from build123d import *

# Parameters (mm, degrees)
SKETCH_W     = 72
SKETCH_H     = 72
PAD_DEPTH    = 1.5
PAD001_DEPTH = 6
SKETCH002_R  = 1.6
POCKET_DEPTH = 7.501
FILLET_R     = 2
CHAMFER_SIZE = 1


with BuildPart() as part:
    # Sketch → Pad (new body)
    with BuildSketch(Plane.XY):
        with Locations((36, -36)):
            Rectangle(SKETCH_W, SKETCH_H)
    extrude(amount=PAD_DEPTH)

    # Sketch001 (on Face6 of Pad) → Pad001 (join)
    with BuildSketch(Plane.XY.offset(1.5)):
        with BuildLine():
            ThreePointArc((0, -8), (5.656854, -5.656854), (8, 0))
            Line((0, 0), (8, 0))
            Line((0, -8), (0, 0))
        make_face()
        with BuildLine():
            ThreePointArc((8, -72), (5.656854, -66.343146), (0, -64))
            Line((0, -72), (0, -64))
            Line((8, -72), (0, -72))
        make_face()
        with BuildLine():
            ThreePointArc((72, -64), (66.343146, -66.343146), (64, -72))
            Line((64, -72), (72, -72))
            Line((72, -72), (72, -64))
        make_face()
        with BuildLine():
            ThreePointArc((64, 0), (66.343146, -5.656854), (72, -8))
            Line((72, -8), (72, 0))
            Line((72, 0), (64, 0))
        make_face()
    extrude(amount=PAD001_DEPTH)

    # Sketch002 (on Face14 of Pad001) → Pocket (cut, through all)
    with BuildSketch(Plane.XY.offset(7.5)):
        with Locations((4, -4)):
            Circle(SKETCH002_R)
        with Locations((68, -4)):
            Circle(SKETCH002_R)
        with Locations((68, -68)):
            Circle(SKETCH002_R)
        with Locations((4, -68)):
            Circle(SKETCH002_R)
    extrude(amount=-POCKET_DEPTH, mode=Mode.SUBTRACT)

    # Fillet
    fillet_edges = [part.edges().sort_by_distance(p)[0] for p in [
        (0, 0, 4.5),
        (72, 0, 4.5),
        (0, -72, 4.5),
        (72, -72, 4.5),
    ]]
    fillet(fillet_edges, radius=FILLET_R)

    # Chamfer
    chamfer_edges = [part.edges().sort_by_distance(p)[0] for p in [
        (36, -72, 0),
    ]]
    chamfer(chamfer_edges, length=CHAMFER_SIZE)


solid = part.part
Could you check a few things on this model? Use its own coordinates, in mm. A direction names the side the tool comes from. Give positions to 0.01 mm unless a question says otherwise; leave off trailing zeros. Order: outer loops, then holes, each group sorted by start corner. A loop starts at its lowest first (then second) coordinate and runs counter-clockwise, first axis right, second up.
1. Suppose I cut it at B-B (y = -68). List the corners of the cut face in (x, z) for me, plus the area to 3 significant figures.
2. Will these pins go through, and if not, where does the flat tip stop? P1, Ø2, axis at x = 14.5, y = -27.5, coming from the +Z side; P2, Ø3.5, axis at x = 4, y = -4, coming from the +Z side.
3. I need wall thicknesses on L1, parallel to Y at x = 4, z = 3.75; L2, parallel to Z at x = 22.5, y = -27; L3, parallel to X at y = -6, z = 3. Which ranges of each line are inside material? Lowest first, please.
4. Suppose I cut it at C-C (y = -55.5). List the corners of the cut face in (x, z) for me, plus the area to 3 significant figures.
5. Suppose I cut it at A-A (x = 4). List the corners of the cut face in (y, z) for me.
6. We'd pull the mould along X, two halves only. Please class faces 3 (the cylindrical face through (69.526, -67.519, 3.802)), 4 (the conical face through (1, -70.98, 0.4)), 5 (the flat face through (3, -70, 7.5)): pulls with the +X half, pulls with the -X half, needs draft (parallel to the pull), parting line crosses it, or undercut.
7. Suppose I cut it at D-D (x = 34). List the corners of the cut face in (y, z) for me.
8. For faces 1 (the cylindrical face through (4.86, -2.65, 3.8)), 2 (the flat face through (35, -35, 1.5)), which set-ups out of +Z, -Z, +X, -X, +Y, -Y let a thin tool reach every point of the face, with its end or its side?
Solved:
1. outline: (0, 1) - (1, 0) - (2.4, 0) - (2.4, 7.5) - (0, 7.5) - close; (5.6, 0) - (66.4, 0) - (66.4, 7.5) - (65.07, 7.5) - (65.07, 1.5) - (6.93, 1.5) - (6.93, 7.5) - (5.6, 7.5) - close; (69.6, 0) - (71, 0) - (72, 1) - (72, 7.5) - (69.6, 7.5) - close
1. area: 142 mm2
2. P1: stops at z = 1.5
2. P2: stops at z = 7.5
3. L1: y = -72 to -69.6, -66.4 to -65.07, -6.93 to -5.6, -2.4 to 0
3. L2: z = 0 to 1.5
3. L3: x = 0 to 5.29, 66.71 to 72
4. outline: (0, 1) - (1, 0) - (71, 0) - (72, 1) - (72, 1.5) - (0, 1.5) - close
4. area: 107 mm2
5. outline: (-72, 1) - (-71, 0) - (-69.6, 0) - (-69.6, 7.5) - (-72, 7.5) - close; (-66.4, 0) - (-5.6, 0) - (-5.6, 7.5) - (-6.93, 7.5) - (-6.93, 1.5) - (-65.07, 1.5) - (-65.07, 7.5) - (-66.4, 7.5) - close; (-2.4, 0) - (-1, 0) - (0, 1) - (0, 7.5) - (-2.4, 7.5) - close
6. face 3: undercut
6. face 4: pulls with the -X half
6. face 5: needs draft
7. outline: (-72, 1) - (-71, 0) - (-1, 0) - (0, 1) - (0, 1.5) - (-72, 1.5) - close
8. face 1: +Z, -Z
8. face 2: +Z
